The listing builds one solid part. Answer for the finished solid, in the listing's coordinates (mm). Face numbers are marked on the shaded views. A direction names the side the tool comes from. Round coordinates to 2 decimals unless told otherwise and drop trailing zeros. Write each loop counter-clockwise with the first axis right and the second up, starting at its lowest first coordinate (ties: lowest second). Pieces come first, ordered by that corner, then holes. Notation, with made-up numbers: M 24,-3 L 66,-3 A26 cw 66,14 Z; hole C 79.25,41 d3. An arc over 180 degrees is marked long. One line per item, written item: value. Start each with the question number.
(1) Given P1, Ø5, axis at x = -7.5, z = 5, coming from the -Y side; P2, Ø6, axis at x = 2, z = 0, coming from the +Y side; P3, Ø1.2, axis at x = -0.5, y = 1, coming from the +Z side (3 decimals); P4, Ø2, axis at x = -0.5, y = 3, coming from the -Z side (3 decimals), each flat-ended and moving along its own axis, determine where each tip first touches the part or whether it passes through.
(2) For a pull along Z with two mould halves and no side action, classify the marked faces 1, 2 and 3 as released by +Z, released by -Z, zero draft, split by the parting line, or undercut.
(3) Section D-D (y = -1) is taken. Determine the outline of the cut face in (x, z) (3 decimals).
(4) Section A-A (y = 2.25) is taken. Determine the outline of the cut face in (x, z) (3 decimals), plus the area to 3 significant figures.
(5) Consider probe 1 along Z at (x, y) = (3, 1) (3 decimals); probe 2 along Z at (x, y) = (-4, 3.75); probe 3 along X at (y, z) = (-1, -2). Determine where each line is inside the solid, lowest interval first.
(6) For the marked faces 4, 5 and 6, determine the directions among +Z, -Z, +X, -X, +Y, -Y from which every point of the face is accessible in a straight line to the end or side of a thin tool.
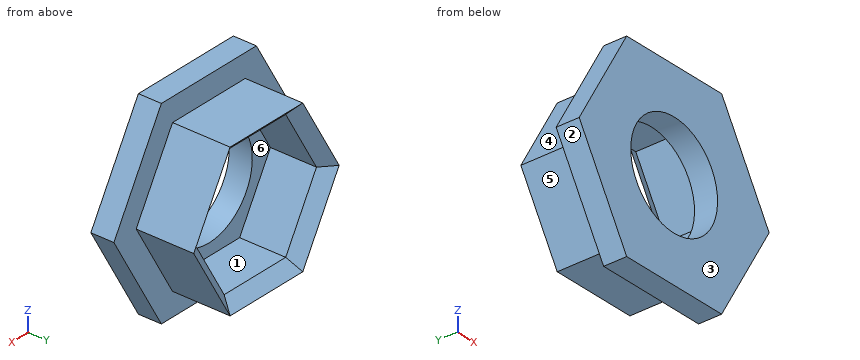
```python
from build123d import *

# Parameters (mm, degrees)
SKETCH2_R           = 4.5
BOSS_EXTRUDE1_DEPTH = 2
BOSS_EXTRUDE2_DEPTH = 5
CHAMFER1_SIZE       = 1


with BuildPart() as part:
    # Sketch2 → Boss-Extrude1 (new body)
    with BuildSketch(Plane.XZ):
        Polygon((-4.921911045, -8.525), (4.921911045, -8.525), (9.84382209, 0), (4.921911045, 8.525), (-4.921911045, 8.525), (-9.84382209, 0), align=None)
        with Locations(Location((0, 0, 0), (0, 0, 270))):
            Circle(SKETCH2_R, mode=Mode.SUBTRACT)
    extrude(amount=BOSS_EXTRUDE1_DEPTH)

    # Sketch3 → Boss-Extrude2 (add)
    with BuildSketch(Plane.XZ):
        Polygon((7.534421013, 0), (3.767210506, 6.525), (-3.767210506, 6.525), (-7.534421013, 0), (-3.767210506, -6.525), (3.767210506, -6.525), align=None)
        Polygon((3.189860237, 5.525), (-3.189860237, 5.525), (-6.379720475, 0), (-3.189860237, -5.525), (3.189860237, -5.525), (6.379720475, 0), align=None, mode=Mode.SUBTRACT)
    extrude(amount=-BOSS_EXTRUDE2_DEPTH)

    # Chamfer1
    chamfer1_edges = [part.edges().sort_by_distance(p)[0] for p in [
        (4.784790356, 5, -2.7625),
        (4.784790356, 5, 2.7625),
        (0, 5, 5.525),
        (-4.784790356, 5, 2.7625),
        (-4.784790356, 5, -2.7625),
        (0, 5, -5.525),
    ]]
    chamfer(chamfer1_edges, length=CHAMFER1_SIZE - 0.0001)  # a hair under: the kernel refuses the full size


solid = part.part
```
Recorded:
1. P1: stops at y = -2
1. P2: stops at y = 0
1. P3: stops at z = 6.525
1. P4: stops at z = -6.525
2. face 1: undercut
2. face 2: released by -Z
2. face 3: zero draft
3. outline: M -9.844,0 L -4.922,-8.525 L 4.922,-8.525 L 9.844,0 L 4.922,8.525 L -4.922,8.525 Z; hole C 0,0 d9
4. outline: M -7.534,0 L -3.767,-6.525 L 3.767,-6.525 L 7.534,0 L 3.767,6.525 L -3.767,6.525 Z; hole M -6.38,0 L -3.19,-5.525 L 3.19,-5.525 L 6.38,0 L 3.19,5.525 L -3.19,5.525 Z
4. area: 41.7 mm2
5. probe 1: z = -6.525 to -5.525, 5.525 to 6.525
5. probe 2: z = -6.12 to -4.12, 4.12 to 6.12
5. probe 3: x = -8.69 to -4.03, 4.03 to 8.69
6. face 4: +Z, -X, +Y
6. face 5: -Z, -X, +Y
6. face 6: +Y
